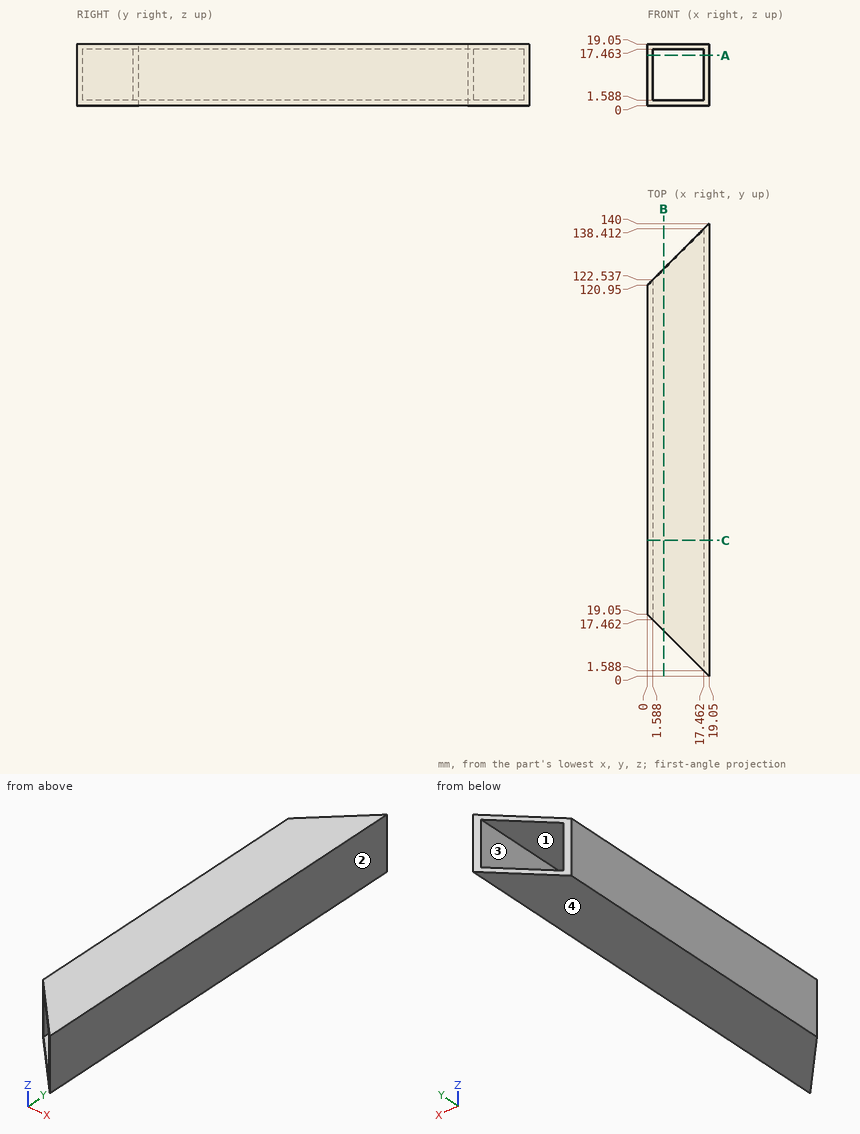
Can you work these out from the drawing? Everything is in mm from the part's minimum corner. Give positions to 0.01 mm unless a question says otherwise; leave off trailing zeros. Loops run counter-clockwise (first coordinate to the right, second up) from the corner with the lowest first, then second, coordinate; pieces in that order, holes last. Notation, with made-up numbers: (0, -25.75) -> (32, -25.75) arc R26 cw to (32, 13.25) -> close; hole circle Ø9 at (-29, -2.5). An arc over 180 degrees is marked (long way). Return JSON: item names as keys, results as strings.
Q1. I want a section at C-C, the plane y = 42. List the corners of the cut face in (x, z) for me.
Checks:
{"outline": "(0, 0) -> (19.05, 0) -> (19.05, 19.05) -> (0, 19.05) -> close; hole (1.59, 1.59) -> (17.46, 1.59) -> (17.46, 17.46) -> (1.59, 17.46) -> close"}
Q2. I want a section at A-A, the plane z = 15.5. List the corners of the cut face in (x, y) for me.
Checks:
{"outline": "(0, 19.05) -> (1.59, 17.46) -> (1.59, 122.54) -> (0, 120.95) -> close; (17.46, 1.59) -> (19.05, 0) -> (19.05, 140) -> (17.46, 138.41) -> close"}
Q3. I want a section at B-B, the plane x = 5. List the corners of the cut face in (y, z) for me.
Checks:
{"outline": "(14.05, 0) -> (125.95, 0) -> (125.95, 1.59) -> (14.05, 1.59) -> close; (14.05, 17.46) -> (125.95, 17.46) -> (125.95, 19.05) -> (14.05, 19.05) -> close"}
Q4. I need wall thicknesses on probe 1 along Z at (x, y) = (16.5, 71); probe 2 along X at (y, z) = (9, 2.75). Which ranges of each line are inside material? Lowest first, please.
Checks:
{"probe 1": "z = 0 to 1.59, 17.46 to 19.05", "probe 2": "x = 17.46 to 19.05"}
Q5. We'd pull the mould along X, two halves only. Please class the marked faces 1, 2, 3 and 4: released by +X, released by -X, zero draft, split by the parting line, or undercut.
Checks:
{"face 1": "undercut", "face 2": "released by +X", "face 3": "undercut", "face 4": "zero draft"}
Q6. For pin 1 Ø10 at (x, z) = (8.5, 2) entering from +Y, with a flat end and sliding along its axis, tell me the tip position at first contact or that it passes through.
Checks:
{"pin 1": "stops at y = 134.43"}
